Check sheet for the modelled part. Datum: model origin and axes. Units: mm. A direction names the side the tool comes from. Round coordinates to 2 decimals unless told otherwise and drop trailing zeros. Order: outer loops, then holes, each group sorted by start corner. A loop starts at its lowest first (then second) coordinate and runs counter-clockwise, first axis right, second up.
from build123d import *

# Parameters (mm, degrees)
ESQUISSE1_R             = 4
BASE_EXTRUSION_DEPTH    = 120
ESQUISSE2_R             = 4
ESQUISSE2_R_2           = 3
ENL_V_MAT_EXTRU_1_DEPTH = 4
ENL_V_START             = -4
ESQUISSE3_R             = 4
ESQUISSE3_R_2           = 3
ENL_V_MAT_EXTRU_2_DEPTH = 4
PER_AGE1_D              = 2.5
PER_AGE1_DEPTH          = 11
PER_AGE1_CBORE_D        = 3
PER_AGE1_CBORE_DEPTH    = 8
PER_AGE1_TIP            = 0.751075774
PER_AGE2_D              = 2.5
PER_AGE2_DEPTH          = 11
PER_AGE2_CBORE_D        = 3
PER_AGE2_CBORE_DEPTH    = 8
PER_AGE2_TIP            = 0.751075774


with BuildPart() as part:
    # Esquisse1 → Base-Extrusion (new body)
    with BuildSketch(Plane.XY):
        Circle(ESQUISSE1_R)
    extrude(amount=BASE_EXTRUSION_DEPTH)

    # Esquisse2 → Enlèv. mat.-Extru.1 (cut)
    with BuildSketch(Plane.XY):
        Circle(ESQUISSE2_R)
        Circle(ESQUISSE2_R_2, mode=Mode.SUBTRACT)
    extrude(amount=ENL_V_MAT_EXTRU_1_DEPTH, mode=Mode.SUBTRACT)

    # Esquisse3 → Enlèv. mat.-Extru.2 (cut)
    with BuildSketch(Plane.XY.offset(120).offset(ENL_V_START)):
        Circle(ESQUISSE3_R)
        Circle(ESQUISSE3_R_2, mode=Mode.SUBTRACT)
    extrude(amount=ENL_V_MAT_EXTRU_2_DEPTH, mode=Mode.SUBTRACT)

    # Perçage1
    with Locations(Plane.XY.offset(120)):
        with Locations((0, 0)):
            CounterBoreHole(PER_AGE1_D / 2, PER_AGE1_CBORE_D / 2, PER_AGE1_CBORE_DEPTH, depth=PER_AGE1_DEPTH)
            with Locations((0, 0, -(PER_AGE1_DEPTH + PER_AGE1_TIP / 2))):  # 118° drill point
                Cone(0, PER_AGE1_D / 2, PER_AGE1_TIP, mode=Mode.SUBTRACT)

    # Perçage2
    with Locations(Plane(origin=(0, 0, 0), x_dir=(-1, 0, 0), z_dir=(0, 0, -1))):
        with Locations((0, 0)):
            CounterBoreHole(PER_AGE2_D / 2, PER_AGE2_CBORE_D / 2, PER_AGE2_CBORE_DEPTH, depth=PER_AGE2_DEPTH)
            with Locations((0, 0, -(PER_AGE2_DEPTH + PER_AGE2_TIP / 2))):  # 118° drill point
                Cone(0, PER_AGE2_D / 2, PER_AGE2_TIP, mode=Mode.SUBTRACT)


solid = part.part
1) Scan lines: line 1 (Y direction, x = 0, z = 110.9); line 2 (Z direction, x = -0.5, y = -3); line 3 (X direction, y = -3.5, z = 52.5). Record each from-to range of solid material in increasing order.
2) Gauge pin test, flat ends, axial feed: pin 1 (1.5 mm diameter, centred on x = 1, z = 80.5, fed in from +Y); pin 2 (2 mm diameter, centred on x = 0, y = 0, fed in from -Z); pin 3 (1 mm diameter, centred on y = 1.5, z = 29, fed in from +X). Record the tip position at first contact, or that the pin passes through.
3) Set-up check for faces 4 (the face through (-0.27, -1.22, 9.52)), 5 (the face through (-0.867, -3.905, 59.216)), 6 (the face through (0.27, -1.22, 110.48)): record each of +Z, -Z, +X, -X, +Y, -Y from which the full face is reachable in a straight line by a thin tool's end or side.
4) Draft check along X on faces 1 (the face through (1, 3, 4)), 2 (the face through (-3, 0, 118)), 3 (the face through (0.05, -0.21, 11.62)). Enter one of: pulls with the +X half, pulls with the -X half, needs draft (parallel to the pull), parting line crosses it, or undercut.
5) Sectioned sample at A-A on z = 45. Record the cut outline in (x, y).
Values found:
1. line 1: y = -4 to -1.25, 1.25 to 4
1. line 2: z = 4 to 116
1. line 3: x = -1.94 to 1.94
2. pin 1: stops at y = 3.99
2. pin 2: stops at z = 11.15
2. pin 3: stops at x = 3.87
3. face 4: -Z
3. face 5: +Z, -Z
3. face 6: +Z
4. face 1: needs draft
4. face 2: parting line crosses it
4. face 3: undercut
5. outline: circle Ø8 at (0, 0)
